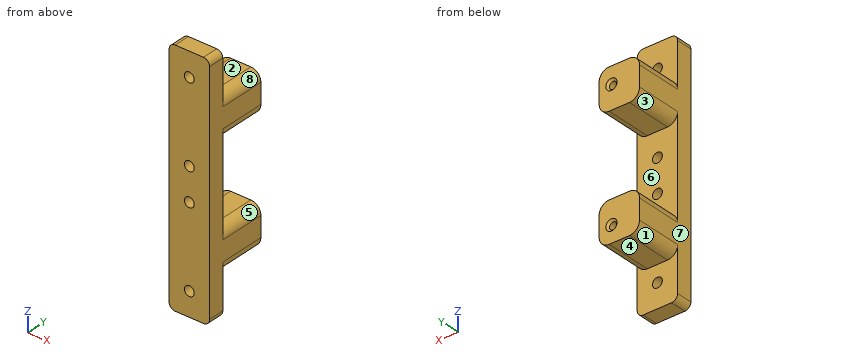
```python
from build123d import *

# Parameters (mm, degrees)
SKETCH1_W                = 10
SKETCH1_H                = 60
BOSS_EXTRUDE1_DEPTH      = 4
F_2_CLEARANCE_HOLE1_D    = 2.4384
FILLET1_R                = 1.5
SKETCH4_W                = 10
SKETCH4_H                = 10
BOSS_EXTRUDE2_DEPTH      = 11.5
FILLET2_R                = 2.5
CHAMFER1_SIZE            = 0.5
FILLET2_OF_MIRROR1_R     = 2.5
CHAMFER1_OF_MIRROR1_SIZE = 0.5


with BuildPart() as part:
    # Sketch1 → Boss-Extrude1 (new body)
    with BuildSketch(Plane(origin=(0, 0, 0), x_dir=(1, 0, 0), z_dir=(0, 1, 0))):
        Rectangle(SKETCH1_W, SKETCH1_H)
    extrude(amount=BOSS_EXTRUDE1_DEPTH)

    # #2 Clearance Hole1 (through all)
    with Locations(Plane(origin=(0, 4, 0), x_dir=(1, 0, 0), z_dir=(0, 1, 0))):
        with Locations((0, -4.08), (0, 24.08), (0, 4.08), (0, -24.08)):
            Hole(F_2_CLEARANCE_HOLE1_D / 2)

    # Fillet1
    fillet1_edges = [part.edges().sort_by_distance(p)[0] for p in [
        (5, 2, 30),
        (-5, 2, 30),
        (-5, 2, -30),
        (5, 2, -30),
    ]]
    fillet(fillet1_edges, radius=FILLET1_R)

    # Sketch4 → Boss-Extrude2 (add)
    with BuildSketch(Plane(origin=(0, 4, 0), x_dir=(1, 0, 0), z_dir=(0, 1, 0))):
        with Locations((0, -15)):
            Rectangle(SKETCH4_W, SKETCH4_H)
    boss_extrude2 = extrude(amount=BOSS_EXTRUDE2_DEPTH)

    # Fillet2
    fillet2_edges = [part.edges().sort_by_distance(p)[0] for p in [
        (-5, 9.75, 10),
        (-5, 9.75, 20),
        (5, 9.75, 20),
        (5, 9.75, 10),
    ]]
    fillet(fillet2_edges, radius=FILLET2_R)

    # Sketch6 → Tap Drill for #2-56 Tap1 (revolve, cut)
    with BuildSketch(Plane(origin=(1.95, 15.5, 15.84), x_dir=(0, 0, 1), z_dir=(1, 0, 0))):
        Polygon((0, 0), (0, 10.69416509), (0.889, 10.16), (0.889, 0), align=None)
    tap_drill_for_2_56_tap1 = revolve(axis=Axis((1.95, 21.85, 15.84), (0, -1, 0)), mode=Mode.SUBTRACT)

    # Chamfer1
    chamfer1_edges = [part.edges().sort_by_distance(p)[0] for p in [
        (1.95, 15.5, 14.951),
    ]]
    chamfer(chamfer1_edges, length=CHAMFER1_SIZE)

    # Mirror1: Boss-Extrude2, Tap Drill for #2-56 Tap1 across plane
    add(boss_extrude2.mirror(Plane.XY))
    add(tap_drill_for_2_56_tap1.mirror(Plane.XY), mode=Mode.SUBTRACT)

    # Fillet2 of Mirror1
    fillet2_of_mirror1_edges = [part.edges().sort_by_distance(p)[0] for p in [
        (-5, 9.75, -10),
        (-5, 9.75, -20),
        (5, 9.75, -20),
        (5, 9.75, -10),
    ]]
    fillet(fillet2_of_mirror1_edges, radius=FILLET2_OF_MIRROR1_R)

    # Chamfer1 of Mirror1
    chamfer1_of_mirror1_edges = [part.edges().sort_by_distance(p)[0] for p in [
        (1.95, 15.5, -14.951),
    ]]
    chamfer(chamfer1_of_mirror1_edges, length=CHAMFER1_OF_MIRROR1_SIZE)


solid = part.part
```
The listing builds one solid part. Answer for the finished solid, in the listing's coordinates (mm). Face numbers are marked on the shaded views. A direction names the side the tool comes from. Give positions to 0.01 mm unless a question says otherwise; leave off trailing zeros. Order: outer loops, then holes, each group sorted by start corner. A loop starts at its lowest first (then second) coordinate and runs counter-clockwise, first axis right, second up. Notation, with made-up numbers: (8.25, -29) -> (23.25, -29) arc R22 ccw to (23.25, -7) -> close; hole circle Ø10 at (-36.5, 19). An arc over 180 degrees is marked (long way). Answer as CSV lines item,"result". Start each with the question number.
Q1. A cutting plane is placed at C-C (x = 0). Determine the outline of the cut face in (y, z), then the cut area to 3 significant figures.
Q2. A cutting plane is placed at A-A (y = 12.75). Determine the outline of the cut face in (x, z).
Q3. Which of the six approach directions +Z, -Z, +X, -X, +Y, -Y give full straight-line access (tool end or side, diameter ignored) to the marked faces 1, 2, 3 and 4?
Q4. A cutting plane is placed at B-B (z = 4.08). Determine the outline of the cut face in (x, y), then the cut area to 3 significant figures.
Q5. Determine the mould class of the marked faces 5, 6, 7 and 8 for opening direction Z: pulls with the +Z half, pulls with the -Z half, needs draft (parallel to the pull), parting line crosses it, or undercut.
Q6. Find the intervals of material crossed by L1, parallel to Z at x = 1.95, y = 12.5; L2, parallel to Z at x = 0, y = 2.3; L3, parallel to Z at x = -0.75, y = 5.25, in increasing order.
Q7. Given pin 1 (3 mm diameter, centred on x = 0, z = -24.08, fed in from +Y); pin 2 (2.5 mm diameter, centred on x = -0.5, y = 11, fed in from -Z); pin 3 (5.5 mm diameter, centred on x = 1, y = 11.5, fed in from +Z), each flat-ended and moving along its own axis, determine where each tip first touches the part or whether it passes through.
Q8. A cutting plane is placed at D-D (y = 1.5). Determine the outline of the cut face in (x, z), then the cut area to 3 significant figures.
Results found:
1,outline,"(0, -30) -> (4, -30) -> (4, -25.3) -> (0, -25.3) -> close; (0, -22.86) -> (4, -22.86) -> (4, -20) -> (15.5, -20) -> (15.5, -10) -> (4, -10) -> (4, -5.3) -> (0, -5.3) -> close; (0, -2.86) -> (4, -2.86) -> (4, 2.86) -> (0, 2.86) -> close; (0, 5.3) -> (4, 5.3) -> (4, 10) -> (15.5, 10) -> (15.5, 20) -> (4, 20) -> (4, 22.86) -> (0, 22.86) -> close; (0, 25.3) -> (4, 25.3) -> (4, 30) -> (0, 30) -> close"
1,area,"431 mm2"
2,outline,"(-5, -17.5) arc R2.5 ccw to (-2.5, -20) -> (2.5, -20) arc R2.5 ccw to (5, -17.5) -> (5, -12.5) arc R2.5 ccw to (2.5, -10) -> (-2.5, -10) arc R2.5 ccw to (-5, -12.5) -> close; (-5, 12.5) arc R2.5 ccw to (-2.5, 10) -> (2.5, 10) arc R2.5 ccw to (5, 12.5) -> (5, 17.5) arc R2.5 ccw to (2.5, 20) -> (-2.5, 20) arc R2.5 ccw to (-5, 17.5) -> close; hole circle Ø1.78 at (1.95, -15.84); hole circle Ø1.78 at (1.95, 15.84)"
3,face 1,"-Z, -X, +Y"
3,face 2,"+Z, +X, -X, +Y"
3,face 3,"-X, +Y"
3,face 4,"-Z, +X, -X, +Y"
4,outline,"(-5, 0) -> (-1.22, 0) -> (-1.22, 4) -> (-5, 4) -> close; (1.22, 0) -> (5, 0) -> (5, 4) -> (1.22, 4) -> close"
4,area,"30.2 mm2"
5,face 5,"undercut"
5,face 6,"undercut"
5,face 7,"needs draft"
5,face 8,"pulls with the +Z half"
6,L1,"-20 to -16.73, -14.95 to -10, 10 to 14.95, 16.73 to 20"
6,L2,"-30 to -25.3, -22.86 to -5.3, -2.86 to 2.86, 5.3 to 22.86, 25.3 to 30"
6,L3,"-20 to -10, 10 to 20"
7,pin 1,"y = 4"
7,pin 2,"z = -20"
7,pin 3,"z = 20"
8,outline,"(-5, -28.5) arc R1.5 ccw to (-3.5, -30) -> (3.5, -30) arc R1.5 ccw to (5, -28.5) -> (5, 28.5) arc R1.5 ccw to (3.5, 30) -> (-3.5, 30) arc R1.5 ccw to (-5, 28.5) -> close; hole circle Ø2.44 at (0, -24.08); hole circle Ø2.44 at (0, -4.08); hole circle Ø2.44 at (0, 4.08); hole circle Ø2.44 at (0, 24.08)"
8,area,"579 mm2"
